Geometry: final body of the model. Coordinates: model frame, mm. Give positions to 0.01 mm unless a question says otherwise; leave off trailing zeros. Write each loop counter-clockwise with the first axis right and the second up, starting at its lowest first coordinate (ties: lowest second). Pieces come first, ordered by that corner, then holes. Notation, with made-up numbers: M 54,68.5 L 62,68.5 A19 ccw 62,88.5 Z; hole C 15.5,70 d3. An arc over 180 degrees is marked long. Use a Markdown table: item, result. Add a question column.
(1) Material intervals for L1, parallel to X at y = 3.4, z = 19.05; L2, parallel to X at y = 2.75, z = 7.5; L3, parallel to Z at x = -43, y = 2.45, sorted ascending.
(2) Cut plane B-B (y = 3.2). State how many separate pieces and enclosed holes the cut face has, plus the area to 3 significant figures.
(3) Draft query along X for faces 1 (the cylindrical face through (-49.947, 2.528, 24.968)), 2 (the flat face through (0, 2, 26)), 3 (the cylindrical face through (-6.3, 2.5, 16.9)). Return one class per face: released by +X, released by -X, zero draft, split by the parting line, or undercut.
(4) Cut plane A-A (z = 20). Output: boundary loops of the cut face in (x, y), plus the area to 3 significant figures.
```python
from build123d import *

# Parameters (mm, degrees)
SKETCH1_W           = 50.8
SKETCH1_H           = 25.4
SKETCH1_R           = 2.15
BOSS_EXTRUDE1_DEPTH = 5
FILLET1_R           = 6.35
FILLET2_R           = 6.35
FILLET3_R           = 0.5


with BuildPart() as part:
    # Sketch1 → Boss-Extrude1 (new body)
    # profile 1 of 2: a face of its own
    with BuildSketch(Plane(origin=(0, 0, 0), x_dir=(1, 0, 0), z_dir=(0, 1, 0))):
        with Locations((-25.4, -12.7)):
            Rectangle(SKETCH1_W, SKETCH1_H)
        with Locations(Location((-44.45, -19.05, 0), (0, 0, 270))):
            Circle(SKETCH1_R, mode=Mode.SUBTRACT)
        with Locations(Location((-6.35, -19.05, 0), (0, 0, 270))):
            Circle(SKETCH1_R, mode=Mode.SUBTRACT)
        with Locations(Location((-6.35, -6.35, 0), (0, 0, 270))):
            Circle(SKETCH1_R, mode=Mode.SUBTRACT)
        with Locations(Location((-44.45, -6.35, 0), (0, 0, 270))):
            Circle(SKETCH1_R, mode=Mode.SUBTRACT)
    # profile 2 of 2: a face of its own
    with BuildSketch(Plane(origin=(0, 0, 0), x_dir=(1, 0, 0), z_dir=(0, 1, 0))):
        Polygon((0, -51.838336263), (0, -25.4), (-50.8, -25.4), (-25.653556262, -40.356808445), (-6.35, -51.838336263), align=None)
        with Locations(Location((-6.35, -44.45, 0), (0, 0, 270))):
            Circle(SKETCH1_R, mode=Mode.SUBTRACT)
    extrude(amount=BOSS_EXTRUDE1_DEPTH)

    # Fillet1
    fillet1_edges = [part.edges().sort_by_distance(p)[0] for p in [
        (0, 2.5, 0),
        (-50.8, 2.5, 0),
        (-50.8, 2.5, 25.4),
        (0, 2.5, 51.838336263),
    ]]
    fillet(fillet1_edges, radius=FILLET1_R - 0.0001)  # a hair under: the kernel refuses the full size

    # Fillet2
    fillet2_edges = [part.edges().sort_by_distance(p)[0] for p in [
        (-6.35, 2.5, 51.838336263),
    ]]
    fillet(fillet2_edges, radius=FILLET2_R - 0.0004)  # a hair under: the kernel refuses the full size

    # Fillet3
    fillet3_edges = [part.edges().sort_by_distance(p)[0] for p in [
        (0, 0, 25.400301661),
        (0, 5, 25.400301661),
        (-25.4, 0, 0),
        (-28.645831614, 0, 38.577038322),
        (-50.8, 0, 14.069262895),
        (-49.969763738, 0, 24.927820308),
        (-48.94015735, 0, 1.85984265),
        (-1.85984265, 0, 1.85984265),
        (-25.4, 5, 0),
        (-50.8, 5, 14.069262895),
        (-28.645831614, 5, 38.577038322),
        (-49.969763738, 5, 24.927820308),
        (-48.94015735, 5, 1.85984265),
        (-1.85984265, 5, 1.85984265),
        (-3.210553792, 0, 49.970106285),
        (-3.210553792, 5, 49.970106285),
    ]]
    fillet(fillet3_edges, radius=FILLET3_R)


solid = part.part
```
Answer list:
| question | item | result |
|---|---|---|
| 1 | L1 | -50.8 to -46.6, -42.3 to -8.5, -4.2 to 0 |
| 1 | L2 | -50.8 to -46.27, -42.63 to -8.17, -4.53 to 0 |
| 1 | L3 | 0 to 4.76, 7.94 to 17.46, 20.64 to 30.04 |
| 2 | separate pieces | 1 |
| 2 | enclosed holes | 5 |
| 2 | area | 1,940 mm² |
| 3 | face 1 | released by -X |
| 3 | face 2 | released by +X |
| 3 | face 3 | undercut |
| 4 | outline | M -50.8,0.5 A0.5 ccw -50.3,0 L -46.38,0 L -46.38,5 L -50.3,5 A0.5 ccw -50.8,4.5 Z; M -42.52,0 L -8.28,0 L -8.28,5 L -42.52,5 Z; M -4.42,0 L -0.5,0 A0.5 ccw 0,0.5 L 0,4.5 A0.5 ccw -0.5,5 L -4.42,5 Z |
| 4 | area | 215 mm² |
